from build123d import *

# Parameters (mm, degrees)
BOSS_EXTRUDE1_DEPTH = 10
BOSS_EXTRUDE2_DEPTH = 10
BOSS_EXTRUDE4_DEPTH = 20
CUT_EXTRUDE3_DEPTH  = 57


with BuildPart() as part:
    # Sketch1 → Boss-Extrude1 (new body)
    with BuildSketch(Plane.XY):
        Polygon((0, 0), (-40, 0), (0, 40), align=None)
    extrude(amount=BOSS_EXTRUDE1_DEPTH)

    # Sketch2 → Boss-Extrude2 (add)
    with BuildSketch(Plane(origin=(0, 0, 0), x_dir=(-1, 0, 0), z_dir=(0, 0, -1))):
        with BuildLine():
            Line((0, 40), (0, 0))
            Line((0, 0), (40, 0))
            ThreePointArc((40, 0), (28.284271247, 28.284271247), (0, 40))
        make_face()
    extrude(amount=BOSS_EXTRUDE2_DEPTH)

    # Sketch3 → Boss-Extrude4 (add)
    with BuildSketch(Plane(origin=(0, 0, -10), x_dir=(-1, 0, 0), z_dir=(0, 0, -1))):
        Polygon((0, 40), (0, 0), (40, 0), align=None)
    extrude(amount=BOSS_EXTRUDE4_DEPTH)

    # Sketch5 → Cut-Extrude3 (cut)
    with BuildSketch(Plane.XZ):
        Polygon((0, -30), (-40, -10), (-40, -30), align=None)
    extrude(amount=-CUT_EXTRUDE3_DEPTH, mode=Mode.SUBTRACT)


solid = part.part
Geometry: final body of the model. Coordinates: model frame, mm. A direction names the side the tool comes from. Give positions to 0.01 mm unless a question says otherwise; leave off trailing zeros. Order: outer loops, then holes, each group sorted by start corner. A loop starts at its lowest first (then second) coordinate and runs counter-clockwise, first axis right, second up. Notation, with made-up numbers: (54, 20) -> (90, 20) arc R27 cw to (90, 50) -> close; hole circle Ø8 at (33.5, 84.25). An arc over 180 degrees is marked (long way). Write each question's results on one line, items separated by ' | '.
1) Cut plane A-A (y = 30). Output: boundary loops of the cut face in (x, z).
Geometry says:
outline: (-26.46, -10) -> (-10, -10) -> (-10, -25) -> (0, -30) -> (0, 10) -> (-10, 10) -> (-10, 0) -> (-26.46, 0) -> close
2) First-contact query: pin 1 Ø1 at (x, y) = (-23, 25) entering from +Z; pin 2 Ø4 at (x, z) = (-11.5, -5) entering from +Y; pin 3 Ø12 at (x, y) = (-18.5, 24.5) entering from -Z. Flat tips, straight axial feed; report the tip coordinate or a pass-through.
Geometry says:
pin 1: stops at z = 0 | pin 2: stops at y = 38.86 | pin 3: stops at z = -23.75
3) Cut plane C-C (z = -15). Output: boundary loops of the cut face in (x, y).
Geometry says:
outline: (-30, 0) -> (0, 0) -> (0, 40) -> (-30, 10) -> close
4) Cut plane B-B (x = -22.5). Output: boundary loops of the cut face in (y, z), and give its area (3 significant figures).
Geometry says:
outline: (0, -18.75) -> (17.5, -18.75) -> (17.5, -10) -> (33.07, -10) -> (33.07, 0) -> (17.5, 0) -> (17.5, 10) -> (0, 10) -> close | area: 659 mm²
5) Set-up query: faces 1 (the face through (-28.594, 27.972, -4.93)), 2 (the face through (-11, 29, -15)), 3 (the face through (-23, 25, 0)). Return all of +Z, -Z, +X, -X, +Y, -Y with unobstructed straight access to the full face (end or side cutting, diameter ignored); none if empty.
Geometry says:
face 1: +Z, -Z, -X, +Y | face 2: -Z, -X, +Y | face 3: +Z, -X, +Y
6) Cut plane D-D (z = -24.5). Output: boundary loops of the cut face in (x, y).
Geometry says:
outline: (-11, 0) -> (0, 0) -> (0, 40) -> (-11, 29) -> close
7) Line query: line 1 along Z through (x, y) = (-27, 16.5); line 2 along Z through (x, y) = (-5.5, 28.5); line 3 along X through (y, z) = (24, -6.5). Output: solid intervals per line, ascending.
Geometry says:
line 1: z = -10 to 0 | line 2: z = -27.25 to 10 | line 3: x = -32 to 0
